Geometry: final body of the model. Coordinates: model frame, mm. A direction names the side the tool comes from. Give positions to 0.01 mm unless a question says otherwise; leave off trailing zeros. Order: outer loops, then holes, each group sorted by start corner. A loop starts at its lowest first (then second) coordinate and runs counter-clockwise, first axis right, second up. Notation, with made-up numbers: (43.5, 53) -> (94.5, 53) arc R19 cw to (94.5, 90) -> close; hole circle Ø11 at (62.25, -24). An arc over 180 degrees is marked (long way). Write item = value, one per line.
```python
from build123d import *

# Parameters (mm, degrees)
SKETCH1_R           = 40
BOSS_EXTRUDE1_DEPTH = 100
SKETCH2_R           = 20
BOSS_EXTRUDE2_DEPTH = 20
FILLET2_R           = 40
SKETCH3_W           = 41.30426334
SKETCH3_H           = 80
CUT_EXTRUDE5_DEPTH  = 80
SKETCH5_R           = 20
CUT_EXTRUDE6_DEPTH  = 10


with BuildPart() as part:
    # Sketch1 → Boss-Extrude1 (new body)
    with BuildSketch(Plane(origin=(0, 0, 0), x_dir=(1, 0, 0), z_dir=(0, 1, 0))):
        with Locations(Location((0, 0, 0), (0, 0, 270))):
            Circle(SKETCH1_R)
    extrude(amount=BOSS_EXTRUDE1_DEPTH)

    # Sketch2 → Boss-Extrude2 (add)
    with BuildSketch(Plane.XZ):
        with Locations(Location((0, 0, 0), (0, 0, 270))):
            Circle(SKETCH2_R)
    extrude(amount=BOSS_EXTRUDE2_DEPTH)

    # Fillet2
    fillet2_edges = [part.edges().sort_by_distance(p)[0] for p in [
        (0, 100, -40),
    ]]
    fillet(fillet2_edges, radius=FILLET2_R)

    # Sketch3 → Cut-Extrude5 (cut)
    with BuildSketch(Plane(origin=(0, 100, 0), x_dir=(1, 0, 0), z_dir=(0, 1, 0))):
        with Locations((20.65213167, 0)):
            Rectangle(SKETCH3_W, SKETCH3_H)
    extrude(amount=-CUT_EXTRUDE5_DEPTH, mode=Mode.SUBTRACT)

    # Sketch5 → Cut-Extrude6 (cut)
    with BuildSketch(Plane(origin=(0, 0, 0), x_dir=(0, 0, -1), z_dir=(1, 0, 0))):
        with Locations((0, 56.442620776)):
            Circle(SKETCH5_R)
    extrude(amount=-CUT_EXTRUDE6_DEPTH, mode=Mode.SUBTRACT)


solid = part.part
```
1) Section query B-B (y = 63). Output: boundary loops of the cut face in (x, z), plus the area to 3 significant figures.
Check sheet entries:
outline = (-10, -18.89) -> (-10, 18.89) -> (0, 18.89) -> (0, 39.89) arc R39.89 ccw to (0, -39.89) -> (0, -18.89) -> close
area = 2,120 mm²
2) Reachability of faces 4 (the face through (0, 69, -17)), 5 (the face through (-19.524, -9.86, 4.336)), 6 (the face through (-4.93, 76.272, 2.604)), 7 (the face through (0, -20, 0)) from +Z, -Z, +X, -X, +Y, -Y: full face, straight path, thin tool, end or side. Return the list, or none.
Check sheet entries:
face_4 = +Z, -Z, +X, +Y
face_5 = -Y
face_6 = +X
face_7 = +Z, -Z, +X, -X, -Y
3) Section query C-C (x = 25). Output: boundary loops of the cut face in (y, z).
Check sheet entries:
outline = (0, -31.22) -> (20, -31.22) -> (20, 31.22) -> (0, 31.22) -> close
4) Line query: line 1 (Y direction, x = 8, z = 28); line 2 (Y direction, x = 3.5, z = -4.5); line 3 (Y direction, x = -3.5, z = 0). Output: solid intervals per line, ascending. Write a range as from..to.
Check sheet entries:
line_1 = 0..20
line_2 = -20..20
line_3 = -20..36.44, 76.44..99.85
5) First-contact query: P1, Ø2, axis at x = -4, y = 4.5, coming from the +Z side; P2, Ø3, axis at x = -11.5, y = -0.5, coming from the -Z side; P3, Ø20, axis at y = 57, z = -4.5, coming from the +X side. Flat tips, straight axial feed; report the tip coordinate or a pass-through.
Check sheet entries:
P1 = 39.89
P2 = -38.71
P3 = -10
6) Section query D-D (z = 8). Output: boundary loops of the cut face in (x, y).
Check sheet entries:
outline = (-39.19, 0) -> (-18.33, 0) -> (-18.33, -20) -> (18.33, -20) -> (18.33, 0) -> (39.19, 0) -> (39.19, 20) -> (0, 20) -> (0, 38.11) -> (-10, 38.11) -> (-10, 74.77) -> (0, 74.77) -> (0, 99.19) arc R39.19 ccw to (-39.19, 60) -> close
7) Mould query, pull axis Y, two halves, no side actions, for faces 1 (the face through (-10, 57, 0)), 2 (the face through (18.3, 0, -9.4)), 3 (the face through (-39.05, 22.91, -8.67)). Classes: +Y half, -Y half, draft (parallel to the pull), parting line (faces both ways), or undercut.
Check sheet entries:
face_1 = undercut
face_2 = -Y half
face_3 = draft
8) Section query A-A (z = 0). Output: boundary loops of the cut face in (x, y), plus the area to 3 significant figures.
Check sheet entries:
outline = (-40, 0) -> (-20, 0) -> (-20, -20) -> (20, -20) -> (20, 0) -> (40, 0) -> (40, 20) -> (0, 20) -> (0, 36.44) -> (-10, 36.44) -> (-10, 76.44) -> (0, 76.44) -> (0, 100) arc R40 ccw to (-40, 60) -> close
area = 4,860 mm²
